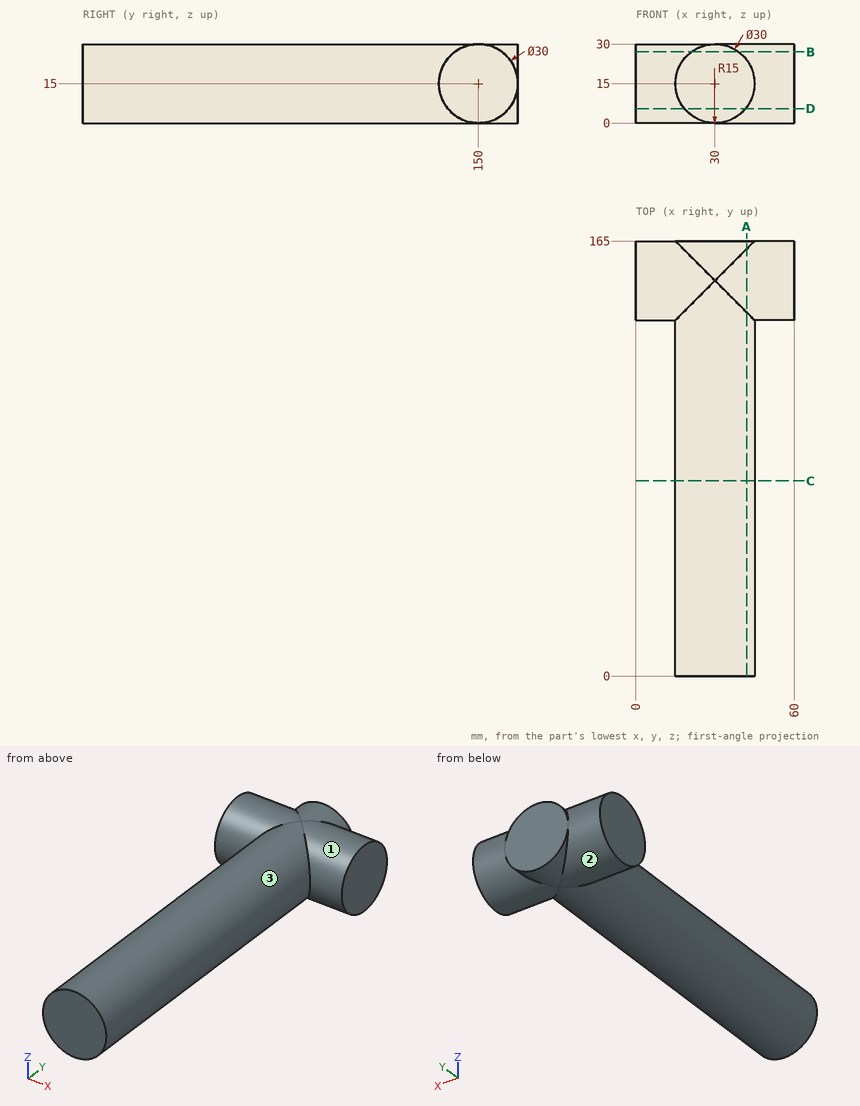
Answer from the drawing. Dimensions are ordinates in mm from the lowest x, y and z of the part. A direction names the side the tool comes from. Coordinates: 2 decimals unless noted, no trailing zeros. Loops run counter-clockwise (first coordinate to the right, second up) from the corner with the lowest first, then second, coordinate; pieces in that order, holes last. Notation, with made-up numbers: (14, 13.5) - (63, 13.5) arc R8 cw to (63, 27.5) - close; hole circle Ø5 at (9.25, 49.25). An arc over 180 degrees is marked (long way). Answer in a Markdown table with one row per item.
1. Straight lines are drawn through the part: line 1 (X direction, y = 23.5, z = 14.75); line 2 (Y direction, x = 50.5, z = 17.75); line 3 (X direction, y = 102, z = 17). For each, find the intervals that lie inside material, in ascending order.
Conclusion:
| item | result |
|---|---|
| line 1 | x = 15 to 45 |
| line 2 | y = 135.25 to 164.75 |
| line 3 | x = 15.13 to 44.87 |
2. Which of the six approach directions +Z, -Z, +X, -X, +Y, -Y give full straight-line access (tool end or side, diameter ignored) to the marked faces 1, 2 and 3?
Conclusion:
| item | result |
|---|---|
| face 1 | +X |
| face 2 | -X |
| face 3 | -Y |
3. Find section C-C, the plane y = 74. Write down the section's boundary in (x, z), then the cut area to 3 significant figures.
Conclusion:
| item | result |
|---|---|
| outline | circle Ø30 at (30, 15) |
| area | 707 mm² |
4. Find section B-B, the plane z = 27. Write down the section's boundary in (x, y).
Conclusion:
| item | result |
|---|---|
| outline | (0, 141) - (21, 141) - (21, 0) - (39, 0) - (39, 141) - (60, 141) - (60, 159) - (39, 159) - (39, 165) - (21, 165) - (21, 159) - (0, 159) - close |
5. Find section A-A, the plane x = 42. Write down the section's boundary in (y, z), then the cut area to 3 significant figures.
Conclusion:
| item | result |
|---|---|
| outline | (0, 6) - (138, 6) arc R15 ccw to (162, 6) - (165, 6) - (165, 24) - (162, 24) arc R15 ccw to (138, 24) - (0, 24) - close |
| area | 3,170 mm² |
6. Find section D-D, the plane z = 5.5. Write down the section's boundary in (x, y), then the cut area to 3 significant figures.
Conclusion:
| item | result |
|---|---|
| outline | (0, 138.39) - (18.39, 138.39) - (18.39, 0) - (41.61, 0) - (41.61, 138.39) - (60, 138.39) - (60, 161.61) - (41.61, 161.61) - (41.61, 165) - (18.39, 165) - (18.39, 161.61) - (0, 161.61) - close |
| area | 4,680 mm² |
7. Given pin 1 (8 mm diameter, centred on x = 44.5, y = 74, fed in from +Z); pin 2 (4 mm diameter, centred on x = 48.5, z = 11, fed in from +Y); pin 3 (3 mm diameter, centred on y = 21.5, z = 26, fed in from -X), each flat-ended and moving along its own axis, determine where each tip first touches the part or whether it passes through.
Conclusion:
| item | result |
|---|---|
| pin 1 | stops at z = 25.71 |
| pin 2 | stops at y = 164.87 |
| pin 3 | stops at x = 18.39 |
